Read the model definition and answer for the solid it produces. Units are mm, in the model's axes. A direction names the side the tool comes from. Round coordinates to 2 decimals unless told otherwise and drop trailing zeros. Order: outer loops, then holes, each group sorted by start corner. A loop starts at its lowest first (then second) coordinate and runs counter-clockwise, first axis right, second up. Notation, with made-up numbers: (68.25, -33.75) - (106.25, -33.75) arc R26 cw to (106.25, 0.25) - close; hole circle Ø8 at (33, 33.25). An arc over 180 degrees is marked (long way). Answer as a JSON object with one key per item and string values. Group by question number.
Q1. Consider line 1 (X direction, y = -6, z = 0.2); line 2 (X direction, y = 10, z = 0.6); line 3 (X direction, y = 2, z = 0.5). Determine where each line is inside the solid, lowest interval first.
Q2. The mould has two halves that part along X. Classify faces 1 (the flat face through (-21.87, 6.3, 0.4)), 2 (the flat face through (6.375, 3.5, 0.4)), 3 (the flat face through (-12.5, 26.38, 0.4)), 4 (the flat face through (-12.675, 3.5, 0.4)): pulls with the +X half, pulls with the -X half, needs draft (parallel to the pull), parting line crosses it, or undercut.
Q3. A cutting plane is placed at B-B on z = 0.2. Determine the outline of the cut face in (x, y) (3 decimals).
Q4. A cutting plane is placed at C-C on x = -10.5. Determine the outline of the cut face in (y, z).
Q5. A cutting plane is placed at D-D on x = 0. Determine the outline of the cut face in (y, z).
Q6. A tool of negligible diameter and unlimited length cuts with its end or side. For faces 5 (the flat face through (-11.204, 23.8, 0.4)), 6 (the flat face through (-17.8, 21.3, 0.4)), 7 (the flat face through (-9.475, 3.5, 0.4)), 8 (the flat face through (-1.8, -4.1, 0.4)), from which of +Z, -Z, +X, -X, +Y, -Y can it reach the whole face along a straight path? Write none if from no direction.
Q7. A cutting plane is placed at A-A on y = 22. Determine the outline of the cut face in (x, z).
Autodesk Inventor part; units mm, degrees
ref_plane "YZ Plane" through (0, 0, 0) normal (1, 0, 0) x (0, 1, 0)
ref_plane "XZ Plane" through (0, 0, 0) normal (0, 1, 0) x (-1, 0, 0)
ref_plane "XY Plane" through (0, 0, 0) normal (0, 0, 1) x (1, 0, 0)
sketch "Sketch1" plane through (0, 0, 0) normal (0, 0, 1) x (1, 0, 0)
  line L0 (-21.87, 21.3003) -> (-21.87, -9.1797)
  line L1 (-21.87, -9.1797) -> (-19.33, -9.1797)
  line L2 (-19.33, -9.1797) -> (-19.33, -4.0997)
  line L3 (-19.33, -4.0997) -> (16.23, -4.0997)
  line L4 (16.23, -4.0997) -> (16.23, -9.1797)
  line L5 (16.23, -9.1797) -> (18.77, -9.1797)
  line L6 (18.77, -9.1797) -> (18.77, 21.3003)
  line L7 (18.77, 21.3003) -> (10.6439, 21.3003)
  line L8 (10.6439, 21.3003) -> (10.6439, 26.3803)
  line L9 (10.6439, 26.3803) -> (8.1039, 26.3803)
  line L10 (8.1039, 26.3803) -> (8.1039, 21.3003)
  line L11 (8.1039, 21.3003) -> (-11.2039, 21.3003)
  line L12 (-11.2039, 21.3003) -> (-11.2039, 26.3803)
  line L13 (-11.2039, 26.3803) -> (-13.7439, 26.3803)
  line L14 (-13.7439, 26.3803) -> (-13.7439, 21.3003)
  line L15 (-13.7439, 21.3003) -> (-21.87, 21.3003)
  dimension "d0" = 40.64
  dimension "d1" = 25.4
  dimension "d2" = 5.08
  dimension "d3" = 2.54
  dimension "d5" = 5.08
  dimension "d18" = 2.54
extrude "Extrusion1" add sketch "Sketch1" along normal blind 0.8255
sketch "Sketch2" plane through (0, 0, 0.8255) normal (0, 0, 1) x (1, 0, 0)
  line L0 (-13.7439, 21.3003) -> (-13.7439, 26.3803)
  arc A0 (-9.4748, 4.1012) -> (-12.6752, 4.1012) centre (-11.075, 8.6003) ccw
  line L1 (-12.6752, 4.1012) -> (-12.6752, 2.8853)
  arc A1 (-12.6752, 2.8853) -> (-9.4748, 2.8853) centre (-11.075, 2.8853) ccw
  line L2 (-9.4748, 2.8853) -> (-9.4748, 4.1012)
  line L3 (-21.87, -9.1797) -> (-21.87, 21.3003)
  point P0 (-19.33, -4.0997)
  dimension "d8" = 5.715
  dimension "d9" = 4.7752
  dimension "d10" = 1.6002
  dimension "d16" = 10.795
  dimension "d17" = 12.7
extrude "Extrusion2" cut sketch "Sketch2" against normal blind 0.8255
pattern_linear "Rectangular Pattern1" count 2 spacing 19.05 along (1, 0, 0) of "Extrusion2"
properties part number "adaptplate"
Result set:
{
 "1": {"line 1": "x = -21.87 to -19.33, 16.23 to 18.77", "line 2": "x = -21.87 to -15.64, -6.51 to 3.41, 12.54 to 18.77", "line 3": "x = -21.87 to -12.41, -9.74 to 6.64, 9.31 to 18.77"},
 "2": {"face 1": "pulls with the -X half", "face 2": "undercut", "face 3": "needs draft", "face 4": "undercut"},
 "3": {"outline": "(-21.87, -9.18) - (-19.33, -9.18) - (-19.33, -4.1) - (16.23, -4.1) - (16.23, -9.18) - (18.77, -9.18) - (18.77, 21.3) - (10.644, 21.3) - (10.644, 26.38) - (8.104, 26.38) - (8.104, 21.3) - (-11.204, 21.3) - (-11.204, 26.38) - (-13.744, 26.38) - (-13.744, 21.3) - (-21.87, 21.3) - close; hole (-12.675, 2.885) arc R1.6 ccw to (-9.475, 2.885) - (-9.475, 4.101) arc R4.775 ccw (long way) to (-12.675, 4.101) - close; hole (6.375, 2.885) arc R1.6 ccw to (9.575, 2.885) - (9.575, 4.101) arc R4.775 ccw (long way) to (6.375, 4.101) - close"},
 "4": {"outline": "(-4.1, 0) - (1.39, 0) - (1.39, 0.83) - (-4.1, 0.83) - close; (13.34, 0) - (21.3, 0) - (21.3, 0.83) - (13.34, 0.83) - close"},
 "5": {"outline": "(-4.1, 0) - (21.3, 0) - (21.3, 0.83) - (-4.1, 0.83) - close"},
 "6": {"face 5": "+Z, -Z, +Y", "face 6": "+Z, -Z, -X, +Y", "face 7": "+Z, -Z", "face 8": "+Z, -Z, -Y"},
 "7": {"outline": "(-13.74, 0) - (-11.2, 0) - (-11.2, 0.83) - (-13.74, 0.83) - close; (8.1, 0) - (10.64, 0) - (10.64, 0.83) - (8.1, 0.83) - close"}
}
